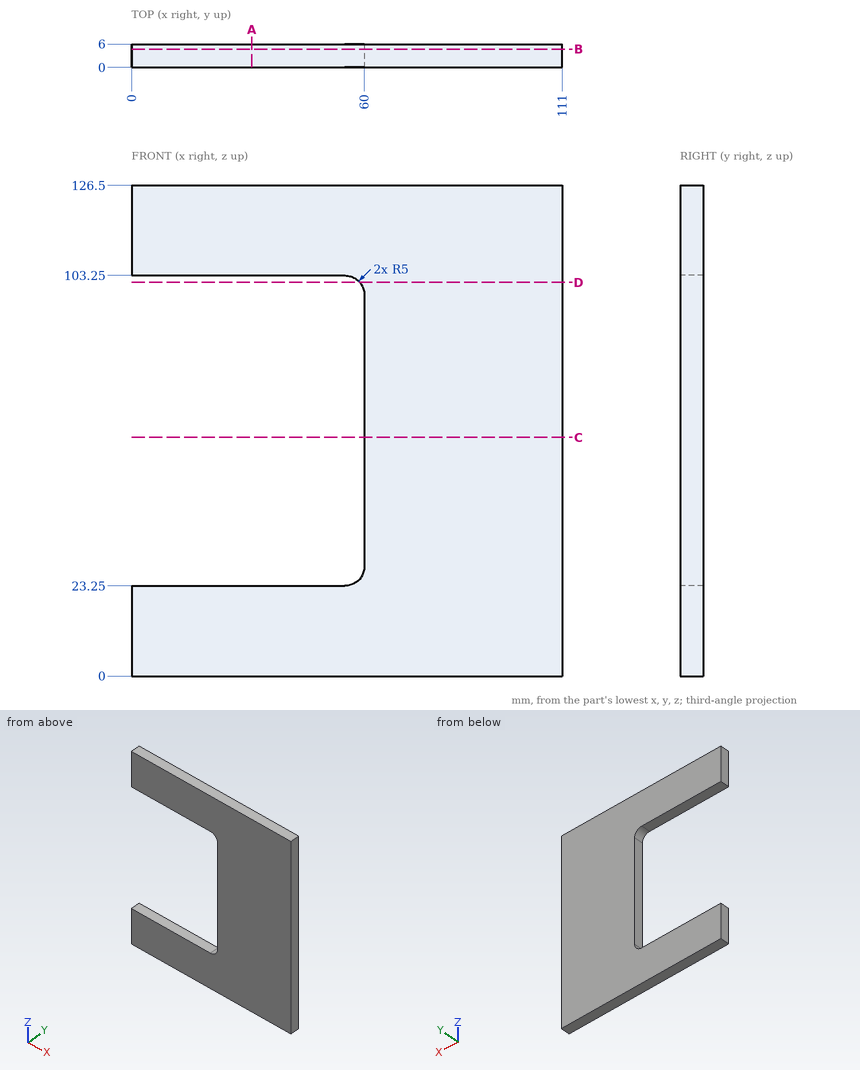
Could you check a few things on this drawing? It's one solid part, dimensions in mm from its lowest x, y, z. Give positions to 0.01 mm unless a question says otherwise; leave off trailing zeros. Order: outer loops, then holes, each group sorted by start corner. A loop starts at its lowest first (then second) coordinate and runs counter-clockwise, first axis right, second up. Notation, with made-up numbers: (-22.5, 51.25) - (-5.5, 51.25) arc R5 ccw to (-5.5, 60.25) - close; hole circle Ø4 at (62.25, 42.25). An arc over 180 degrees is marked (long way). Answer as a JSON object with one key per item and string values. Group by question number.
Item 1: If we section it at A-A on x = 31: Please give me the cut outline in (y, z), and give its area (3 significant figures).
Item 2: For P1, Ø3, axis at y = 1.5, z = 65.5, coming from the -X side, with a flat end and sliding along its axis, tell me the tip position at first contact or that it passes through.
Item 3: Please list where these lines run through material, in increasing order: probe 1 along Z at (x, y) = (49, 3.85); probe 2 along X at (y, z) = (4.2, 39.5); probe 3 along X at (y, z) = (4.4, 99.5).
Item 4: If we section it at D-D on z = 101.5: Please give me the cut outline in (x, y), and give its area (3 significant figures).
Item 5: If we section it at B-B on y = 4.65: Please give me the cut outline in (x, z).
Item 6: If we section it at C-C on z = 61.5: Please give me the cut outline in (x, y).
Result set:
{
 "1": {"outline": "(0, 0) - (6, 0) - (6, 23.25) - (0, 23.25) - close; (0, 103.25) - (6, 103.25) - (6, 126.5) - (0, 126.5) - close", "area": "279 mm²"},
 "2": {"P1": "x = 60"},
 "3": {"probe 1": "0 to 23.25, 103.25 to 126.5", "probe 2": "60 to 111", "probe 3": "59.84 to 111"},
 "4": {"outline": "(58.8, 0) - (111, 0) - (111, 6) - (58.8, 6) - close", "area": "313 mm²"},
 "5": {"outline": "(0, 0) - (111, 0) - (111, 126.5) - (0, 126.5) - (0, 103.25) - (55, 103.25) arc R5 cw to (60, 98.25) - (60, 28.25) arc R5 cw to (55, 23.25) - (0, 23.25) - close"},
 "6": {"outline": "(60, 0) - (111, 0) - (111, 6) - (60, 6) - close"}
}
